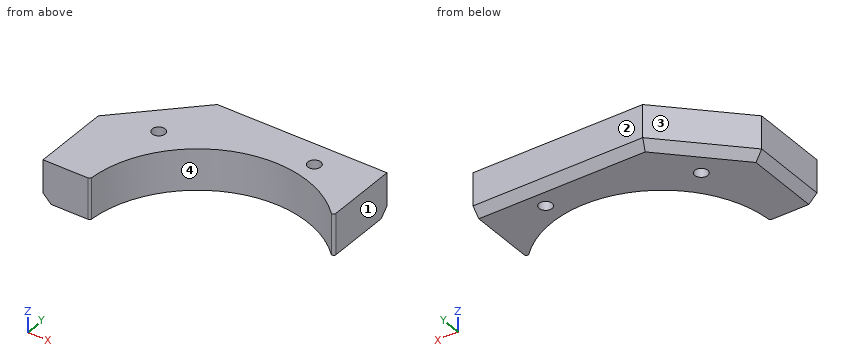
Autodesk Inventor part; units mm, degrees
ref_plane "YZ Plane" through (0, 0, 0) normal (1, 0, 0) x (0, 1, 0)
ref_plane "XZ Plane" through (0, 0, 0) normal (0, 1, 0) x (-1, 0, 0)
ref_plane "XY Plane" through (0, 0, 0) normal (0, 0, 1) x (1, 0, 0)
sketch "Sketch1" plane through (0, 0, 0) normal (0, 0, 1) x (1, 0, 0)
  line L0 (0, 0) -> (58.5, 0)
  line L1 (58.5, 0) -> (58.5, 36)
  line L2 (58.5, 36) -> (0, 36)
  line L3 (0, 36) -> (0, 0)
  dimension "d0" = 58.5
  dimension "d1" = 36
extrude "Extrusion1" add sketch "Sketch1" along normal blind 10
sketch "Sketch2" plane through (0, 0, 10) normal (0, 0, 1) x (1, 0, 0)
  line L0 (0, 0) -> (0, 36)
  line L1 (58.5, 0) -> (0, 0)
  circle A0 centre (38.5, -1) radius 27
  dimension "d6" = 27
  dimension "d7" = 1
  dimension "d8" = 11.5
extrude "Extrusion2" cut sketch "Sketch2" against normal blind 10
sketch "Sketch3" plane through (0, 0, 10) normal (0, 0, 1) x (1, 0, 0)
  line L0 (58.5, 36) -> (58.5, 17.1384)
  line L1 (11.5185, 0) -> (0, 0)
  line L2 (0, 36) -> (58.5, 36)
  point P0 (13, 21.5)
  point P1 (45, 30)
  dimension "d11" = 32
  dimension "d12" = 13.5
  dimension "d13" = 21.5
  dimension "d28" = 6
hole "Hole1" at (13, 21.5, 10) at (45, 30, 10) direction (0, 0, -1) diameter 3.175 depth 10 tip angle 118
chamfer "Chamfer1" distance 17 angle 45 1 edges at (0, 36, 5)
chamfer "Chamfer2" distance 2 angle 45 3 edges at (37.75, 36, 0) (8.5, 27.5, 0) (0, 9.5, 0)
fillet "Fillet1" radius 0.5 2 edges at (58.5, 17.1384, 5) (11.5185, 0, 5)
properties part number "PÁRA-LAMAS DIANTEIRO-ESQ" material "Carbon Steel"
Can you work these out from the model? Positions are in its coordinate system, mm. Face numbers are marked on the shaded views. Round coordinates to 2 decimals unless told otherwise and drop trailing zeros. Loops run counter-clockwise (first coordinate to the right, second up) from the corner with the lowest first, then second, coordinate; pieces in that order, holes last. Notation, with made-up numbers: (55, 38) -> (72, 38) arc R8 cw to (72, 42) -> close; hole circle Ø8 at (68.5, 27.5). An arc over 180 degrees is marked (long way). One line per item, written item: value. Start each with the question number.
1. For pin 1 (1.9 mm diameter, centred on x = 13, y = 21.5, fed in from -Z); pin 2 (4 mm diameter, centred on x = 6.5, z = 2.5, fed in from +Y), each with a flat end and sliding along its axis, tell me the tip position at first contact or that it passes through.
2. If we section it at A-A, the plane y = 21.5: Write out the boundary of the cut face in (x, z).
3. If we section it at C-C, the plane y = 30: Write out the boundary of the cut face in (x, z).
4. If we section it at D-D, the plane z = 3: Write out the boundary of the cut face in (x, y) (1 decimal), then the cut area to 3 significant figures.
5. If we mould it in two halves opening along X, with no side actions, what happens to the marked faces 1, 2, 3 and 4? For each: pulls with the +X half, pulls with the -X half, needs draft (parallel to the pull), parting line crosses it, or undercut.
6. If I drill on probe 1 along X at (y, z) = (21.5, 6.5); probe 2 along X at (y, z) = (30, 2.75); probe 3 along X at (y, z) = (23.5, 7.25), over which ranges is the centre line in solid material (lowest first)?
7. If we section it at B-B, the plane x = 44: Write out the boundary of the cut face in (y, z), then the cut area to 3 significant figures.
Calculated:
1. pin 1: passes through
1. pin 2: stops at y = 27.5
2. outline: (2.5, 2) -> (5.33, 0) -> (11.41, 0) -> (11.41, 10) -> (2.5, 10) -> close; (14.59, 0) -> (23.58, 0) -> (23.58, 10) -> (14.59, 10) -> close; (53.42, 0) -> (58.5, 0) -> (58.5, 10) -> (53.42, 10) -> close
3. outline: (11, 2) -> (13.83, 0) -> (43.41, 0) -> (43.41, 10) -> (11, 10) -> close; (46.59, 0) -> (58.5, 0) -> (58.5, 10) -> (46.59, 10) -> close
4. outline: (0, 0) -> (11, 0) arc R0.5 ccw to (11.5, 0.5) arc R27 cw to (57.6, 18) arc R0.5 ccw to (58.5, 18.4) -> (58.5, 36) -> (17, 36) -> (0, 19) -> close; hole circle Ø3.2 at (13, 21.5); hole circle Ø3.2 at (45, 30)
4. area: 934 mm²
5. face 1: pulls with the +X half
5. face 2: needs draft
5. face 3: pulls with the -X half
5. face 4: undercut
6. probe 1: x = 2.5 to 11.41, 14.59 to 23.58, 53.42 to 58.5
6. probe 2: x = 11 to 43.41, 46.59 to 58.5
6. probe 3: x = 4.5 to 27.15, 49.85 to 58.5
7. outline: (25.43, 0) -> (28.77, 0) -> (28.77, 10) -> (25.43, 10) -> close; (31.23, 0) -> (34, 0) -> (36, 2) -> (36, 10) -> (31.23, 10) -> close
7. area: 79.0 mm²
